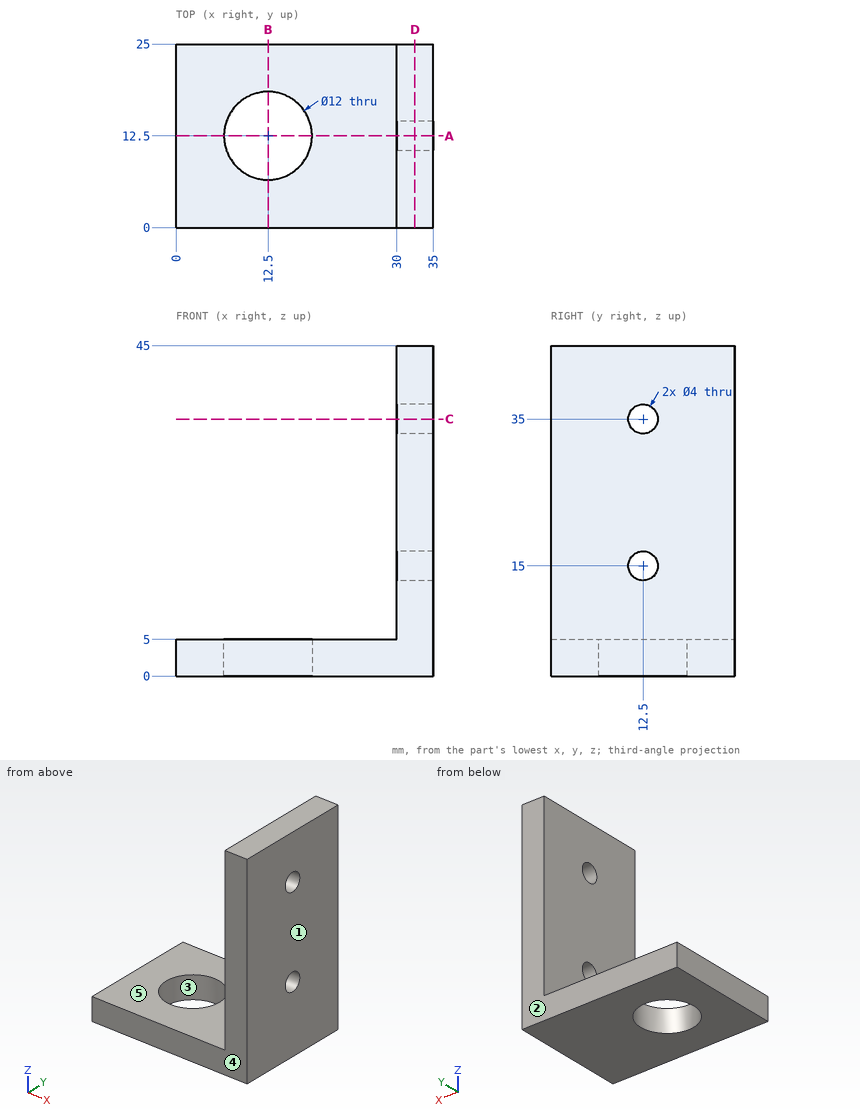
Print and shaded views of the part. All mm, measured from the part's lowest x, y and z. A direction names the side the tool comes from. Round coordinates to 2 decimals unless told otherwise and drop trailing zeros. Write each loop counter-clockwise with the first axis right and the second up, starting at its lowest first coordinate (ties: lowest second). Pieces come first, ordered by that corner, then holes.
Item 1: Two-plate mould, pull along Y, no slides. Class the marked faces 1, 2 and 3: +Y half, -Y half, draft (parallel to the pull), parting line (faces both ways), or undercut.
Results:
face 1: draft
face 2: +Y half
face 3: undercut
Item 2: Which spindle directions (+Z, -Z, +X, -X, +Y, -Y) get a long thin tool onto all of the face, cutting with end or side? Do the marked faces 4 and 5. Say none if no direction does.
Results:
face 4: +Z, -Z, +X, -X, -Y
face 5: +Z, -X, +Y, -Y
Item 3: Cut at D-D, the plane x = 32.5. Give the cut face in (y, z), plus the area to 3 significant figures.
Results:
outline: (0, 0) - (25, 0) - (25, 45) - (0, 45) - close; hole circle Ø4 at (12.5, 15); hole circle Ø4 at (12.5, 35)
area: 1,100 mm2
Item 4: Cut at A-A, the plane y = 12.5. Give the cut face in (x, z).
Results:
outline: (0, 0) - (6.5, 0) - (6.5, 5) - (0, 5) - close; (18.5, 0) - (35, 0) - (35, 13) - (30, 13) - (30, 5) - (18.5, 5) - close; (30, 17) - (35, 17) - (35, 33) - (30, 33) - close; (30, 37) - (35, 37) - (35, 45) - (30, 45) - close
Item 5: Cut at B-B, the plane x = 12.5. Give the cut face in (y, z).
Results:
outline: (0, 0) - (6.5, 0) - (6.5, 5) - (0, 5) - close; (18.5, 0) - (25, 0) - (25, 5) - (18.5, 5) - close
Item 6: Cut at C-C, the plane z = 35. Give the cut face in (x, y), plus the area to 3 significant figures.
Results:
outline: (30, 0) - (35, 0) - (35, 10.5) - (30, 10.5) - close; (30, 14.5) - (35, 14.5) - (35, 25) - (30, 25) - close
area: 105 mm2
Item 7: Drop flat-ended pins along their axis: pin 1 Ø2 at (y, z) = (15.5, 36) entering from -X; pin 2 Ø1.5 at (x, y) = (16, 3) entering from +Z. Give the stop position or say it passes through.
Results:
pin 1: stops at x = 30
pin 2: stops at z = 5
Item 8: Probe L1, parallel to Z at x = 32.65, y = 12.5; L2, parallel to Y at x = 12.5, z = 3.6; L3, parallel to X at y = 9.75, z = 22. List the from-to ranges inside material, lowest first.
Results:
L1: z = 0 to 13, 17 to 33, 37 to 45
L2: y = 0 to 6.5, 18.5 to 25
L3: x = 30 to 35
